from build123d import *

# Parameters (mm, degrees)
SKETCH3_W                = 100
SKETCH3_H                = 100
SKETCH3_W_2              = 80
SKETCH3_H_2              = 80
BOSS_EXTRUDE1_DEPTH      = 120
CUT_EXTRUDE6_DEPTH       = 186.47236991
CIRPATTERN1_COUNT        = 2
CIRPATTERN1_ANGLE        = 90
SKETCH19_R               = 13.375
SKETCH19_R_2             = 8.4375
BOSS_EXTRUDE3_DEPTH      = 10
BOSS_EXTRUDE4_START      = -110
SKETCH19_2_R             = 13.375
SKETCH19_2_R_2           = 8.4375
BOSS_EXTRUDE4_DEPTH      = 10
CUT_EXTRUDE4_DEPTH       = 186.47236991
CUT_EXTRUDE4_DEPTH_BACK  = 186.47236991
SKETCH8_R                = 8.4375
CUT_EXTRUDE11_START      = 120
SKETCH21_R               = 1.5
CUT_EXTRUDE11_DEPTH      = 10
CUT_EXTRUDE12_START      = 10
SKETCH21_2_R             = 1.5
CUT_EXTRUDE12_DEPTH      = 10
SKETCH9_W                = 10
SKETCH9_H                = 80
ELECTRONICSPLATE_DEPTH   = 120
CUT_EXTRUDE10_REACH      = 187.472
SKETCH18_W               = 80
SKETCH18_H               = 100
BEAGLEBONEHOLES_START    = 40
SKETCH12_R               = 1.7
BEAGLEBONEHOLES_DEPTH    = 10
RFDHOLES_START           = 40
SKETCH13_R               = 1.7
RFDHOLES_DEPTH           = 10
ANTENNACAVITY_START      = 30
SKETCH35_W               = 12
SKETCH35_H               = 43
ANTENNACAVITY_DEPTH      = 5
ZIPTIEHOLES_START        = 30
SKETCH36_W               = 3
SKETCH36_H               = 6.5
SKETCH36_W_2             = 6.5
SKETCH36_H_2             = 3
ZIPTIEHOLES_DEPTH        = 10
CUT_EXTRUDE16_START      = 30
SKETCH36_3_W             = 17
SKETCH36_3_H             = 6.5
SKETCH36_3_W_2           = 6.5
SKETCH36_3_H_2           = 15
CUT_EXTRUDE16_DEPTH      = 5
WIREHOLES_START          = 40
SKETCH37_W               = 10
SKETCH37_H               = 10
WIREHOLES_DEPTH          = 10
CUT_EXTRUDE17_DEPTH      = 186.47236991
CUT_EXTRUDE17_DEPTH_BACK = 186.47236991
SKETCH39_W               = 30
SKETCH39_H               = 100
SKETCH39_W_2             = 60
SKETCH39_W_3             = 10
SKETCH39_H_2             = 10


with BuildPart() as part:
    # Sketch3 → Boss-Extrude1 (new body)
    with BuildSketch(Plane(origin=(0, 0, 0), x_dir=(1, 0, 0), z_dir=(0, 1, 0))):
        with Locations((50, 50)):
            Rectangle(SKETCH3_W, SKETCH3_H)
        with Locations((50, 50)):
            Rectangle(SKETCH3_W_2, SKETCH3_H_2, mode=Mode.SUBTRACT)
    extrude(amount=BOSS_EXTRUDE1_DEPTH)

    # Sketch6 → Cut-Extrude6 (cut, symmetric)
    with BuildSketch(Plane.XY):
        Polygon((14.84187473, 110), (50, 67.810249676), (85.15812527, 110), align=None)
        Polygon((56.508541397, 60), (90, 100.189750324), (90, 19.810249676), align=None)
        Polygon((14.84187473, 10), (50, 52.189750324), (85.15812527, 10), align=None)
        Polygon((10, 19.810249676), (43.491458603, 60), (10, 100.189750324), align=None)
    cut_extrude6 = extrude(amount=CUT_EXTRUDE6_DEPTH, both=True, mode=Mode.SUBTRACT)

    # CirPattern1: Cut-Extrude6 ×2 about axis
    cirpattern1_axis = Axis((50, 0, -50), (0, 1, 0))
    for i in range(1, CIRPATTERN1_COUNT):
        add(cut_extrude6.rotate(cirpattern1_axis, i * CIRPATTERN1_ANGLE / (CIRPATTERN1_COUNT - 1)), mode=Mode.SUBTRACT)

    # Sketch19 → Boss-Extrude3 (add)
    # profile 1 of 4: a face of its own
    with BuildSketch(Plane(origin=(0, 120, 0), x_dir=(1, 0, 0), z_dir=(0, 1, 0))):
        with Locations((13.375, 86.625)):
            Circle(SKETCH19_R)
        with Locations((13.375, 86.625)):
            Circle(SKETCH19_R_2, mode=Mode.SUBTRACT)
    # profile 2 of 4: a face of its own
    with BuildSketch(Plane(origin=(0, 120, 0), x_dir=(1, 0, 0), z_dir=(0, 1, 0))):
        with Locations((86.625, 86.625)):
            Circle(SKETCH19_R)
        with Locations((86.625, 86.625)):
            Circle(SKETCH19_R_2, mode=Mode.SUBTRACT)
    # profile 3 of 4: a face of its own
    with BuildSketch(Plane(origin=(0, 120, 0), x_dir=(1, 0, 0), z_dir=(0, 1, 0))):
        with Locations((86.625, 13.375)):
            Circle(SKETCH19_R)
        with Locations((86.625, 13.375)):
            Circle(SKETCH19_R_2, mode=Mode.SUBTRACT)
    # profile 4 of 4: a face of its own
    with BuildSketch(Plane(origin=(0, 120, 0), x_dir=(1, 0, 0), z_dir=(0, 1, 0))):
        with Locations((13.375, 13.375)):
            Circle(SKETCH19_R)
        with Locations((13.375, 13.375)):
            Circle(SKETCH19_R_2, mode=Mode.SUBTRACT)
    extrude(amount=-BOSS_EXTRUDE3_DEPTH)

    # Sketch19<2> → Boss-Extrude4 (add)
    # profile 1 of 4: a face of its own
    with BuildSketch(Plane(origin=(0, 120, 0), x_dir=(1, 0, 0), z_dir=(0, 1, 0)).offset(BOSS_EXTRUDE4_START)):
        with Locations((13.375, 86.625)):
            Circle(SKETCH19_2_R)
    # profile 2 of 4: a face of its own
    with BuildSketch(Plane(origin=(0, 120, 0), x_dir=(1, 0, 0), z_dir=(0, 1, 0)).offset(BOSS_EXTRUDE4_START)):
        with Locations((86.625, 86.625)):
            Circle(SKETCH19_2_R)
        with Locations((86.625, 86.625)):
            Circle(SKETCH19_2_R_2, mode=Mode.SUBTRACT)
    # profile 3 of 4: a face of its own
    with BuildSketch(Plane(origin=(0, 120, 0), x_dir=(1, 0, 0), z_dir=(0, 1, 0)).offset(BOSS_EXTRUDE4_START)):
        with Locations((86.625, 13.375)):
            Circle(SKETCH19_2_R)
        with Locations((86.625, 13.375)):
            Circle(SKETCH19_2_R_2, mode=Mode.SUBTRACT)
    # profile 4 of 4: a face of its own
    with BuildSketch(Plane(origin=(0, 120, 0), x_dir=(1, 0, 0), z_dir=(0, 1, 0)).offset(BOSS_EXTRUDE4_START)):
        with Locations((13.375, 13.375)):
            Circle(SKETCH19_2_R)
        with Locations((13.375, 13.375)):
            Circle(SKETCH19_2_R_2, mode=Mode.SUBTRACT)
    extrude(amount=-BOSS_EXTRUDE4_DEPTH)

    # Sketch8 → Cut-Extrude4 (cut, two sides: drawn at the far end of the back side and taken through both)
    with BuildSketch(Plane(origin=(0, 0, 0), x_dir=(1, 0, 0), z_dir=(0, 1, 0)).offset(-CUT_EXTRUDE4_DEPTH_BACK)):
        with Locations(Location((13.375, 86.625, 0), (0, 0, 90))):
            Circle(SKETCH8_R)
        with Locations(Location((86.625, 86.625, 0), (0, 0, 90))):
            Circle(SKETCH8_R)
        with Locations(Location((13.375, 13.375, 0), (0, 0, 90))):
            Circle(SKETCH8_R)
        with Locations(Location((86.625, 13.375, 0), (0, 0, 90))):
            Circle(SKETCH8_R)
    extrude(amount=CUT_EXTRUDE4_DEPTH + CUT_EXTRUDE4_DEPTH_BACK, mode=Mode.SUBTRACT)

    # Sketch21 → Cut-Extrude11 (cut)
    with BuildSketch(Plane(origin=(0, 0, 0), x_dir=(1, 0, 0), z_dir=(0, 1, 0)).offset(CUT_EXTRUDE11_START)):
        with Locations(Location((5, 50, 0), (0, 0, 270))):
            Circle(SKETCH21_R)
        with Locations(Location((50, 95, 0), (0, 0, 270))):
            Circle(SKETCH21_R)
        with Locations(Location((95, 50, 0), (0, 0, 270))):
            Circle(SKETCH21_R)
        with Locations(Location((50, 5, 0), (0, 0, 270))):
            Circle(SKETCH21_R)
    extrude(amount=-CUT_EXTRUDE11_DEPTH, mode=Mode.SUBTRACT)

    # Sketch21<2> → Cut-Extrude12 (cut)
    with BuildSketch(Plane(origin=(0, 0, 0), x_dir=(1, 0, 0), z_dir=(0, 1, 0)).offset(CUT_EXTRUDE12_START)):
        with Locations(Location((5, 50, 0), (0, 0, 270))):
            Circle(SKETCH21_2_R)
        with Locations(Location((50, 95, 0), (0, 0, 270))):
            Circle(SKETCH21_2_R)
        with Locations(Location((95, 50, 0), (0, 0, 270))):
            Circle(SKETCH21_2_R)
        with Locations(Location((50, 5, 0), (0, 0, 270))):
            Circle(SKETCH21_2_R)
    extrude(amount=-CUT_EXTRUDE12_DEPTH, mode=Mode.SUBTRACT)

    # Sketch9 → ElectronicsPlate (add)
    with BuildSketch(Plane(origin=(0, 0, 0), x_dir=(1, 0, 0), z_dir=(0, 1, 0))):
        with Locations((35, 50)):
            Rectangle(SKETCH9_W, SKETCH9_H)
    extrude(amount=ELECTRONICSPLATE_DEPTH)

    # Sketch18 → Cut-Extrude10 (cut, up to next)
    with BuildSketch(Plane.ZY, mode=Mode.PRIVATE) as cut_extrude10_sk1:
        with Locations((-50, 60)):
            Rectangle(SKETCH18_W, SKETCH18_H)
    cut_extrude10_tool1 = extrude(cut_extrude10_sk1.sketch, amount=-CUT_EXTRUDE10_REACH, mode=Mode.PRIVATE) & part.part
    add(cut_extrude10_tool1.solids().sort_by_distance((0, 60, -50))[0], mode=Mode.SUBTRACT)

    # Sketch12 → BeagleboneHoles (cut)
    with BuildSketch(Plane(origin=(0, 0, 0), x_dir=(0, 0, -1), z_dir=(1, 0, 0)).offset(BEAGLEBONEHOLES_START)):
        with Locations((25.87, 41.96)):
            Circle(SKETCH12_R)
        with Locations((74.13, 41.96)):
            Circle(SKETCH12_R)
        with Locations((29.045, 108)):
            Circle(SKETCH12_R)
        with Locations((70.955, 108)):
            Circle(SKETCH12_R)
    extrude(amount=-BEAGLEBONEHOLES_DEPTH, mode=Mode.SUBTRACT)

    # Sketch13 → RFDHoles (cut)
    with BuildSketch(Plane(origin=(0, 0, 0), x_dir=(0, 0, -1), z_dir=(1, 0, 0)).offset(RFDHOLES_START)):
        with Locations((50, 30)):
            Circle(SKETCH13_R)
        with Locations((37.5, 67)):
            Circle(SKETCH13_R)
        with Locations((62.5, 67)):
            Circle(SKETCH13_R)
    extrude(amount=-RFDHOLES_DEPTH, mode=Mode.SUBTRACT)

    # Sketch35 → AntennaCavity (cut)
    with BuildSketch(Plane(origin=(0, 0, 0), x_dir=(0, 0, -1), z_dir=(1, 0, 0)).offset(ANTENNACAVITY_START)):
        with Locations((24, 68.5)):
            Rectangle(SKETCH35_W, SKETCH35_H)
        Polygon((18, 90), (30, 90), (50, 90), (50, 100), (18, 100), align=None)
        Polygon((50, 100), (50, 90), (70, 90), (82, 90), (82, 100), align=None)
        with Locations((76, 68.5)):
            Rectangle(SKETCH35_W, SKETCH35_H)
    extrude(amount=ANTENNACAVITY_DEPTH, mode=Mode.SUBTRACT)

    # Sketch36 → ZiptieHoles (cut)
    with BuildSketch(Plane(origin=(0, 0, 0), x_dir=(0, 0, -1), z_dir=(1, 0, 0)).offset(ZIPTIEHOLES_START)):
        with Locations((34, 53.701837694)):
            Rectangle(SKETCH36_W, SKETCH36_H)
        with Locations((14, 53.701837694)):
            Rectangle(SKETCH36_W, SKETCH36_H)
        with Locations((34, 76.513807116)):
            Rectangle(SKETCH36_W, SKETCH36_H)
        with Locations((14, 76.513807116)):
            Rectangle(SKETCH36_W, SKETCH36_H)
        with Locations((34.734232458, 86)):
            Rectangle(SKETCH36_W_2, SKETCH36_H_2)
        with Locations((34.734232458, 104)):
            Rectangle(SKETCH36_W_2, SKETCH36_H_2)
        with Locations((65.265767542, 104)):
            Rectangle(SKETCH36_W_2, SKETCH36_H_2)
        with Locations((65.265767542, 86)):
            Rectangle(SKETCH36_W_2, SKETCH36_H_2)
        with Locations((66, 76.513807116)):
            Rectangle(SKETCH36_W, SKETCH36_H)
        with Locations((86, 76.513807116)):
            Rectangle(SKETCH36_W, SKETCH36_H)
        with Locations((86, 53.701837694)):
            Rectangle(SKETCH36_W, SKETCH36_H)
        with Locations((66, 53.701837694)):
            Rectangle(SKETCH36_W, SKETCH36_H)
    extrude(amount=ZIPTIEHOLES_DEPTH, mode=Mode.SUBTRACT)

    # Sketch36<3> → Cut-Extrude16 (cut)
    with BuildSketch(Plane(origin=(0, 0, 0), x_dir=(0, 0, -1), z_dir=(1, 0, 0)).offset(CUT_EXTRUDE16_START)):
        with Locations((24, 76.513807116)):
            Rectangle(SKETCH36_3_W, SKETCH36_3_H)
        with Locations((34.734232458, 95)):
            Rectangle(SKETCH36_3_W_2, SKETCH36_3_H_2)
        with Locations((65.265767542, 95)):
            Rectangle(SKETCH36_3_W_2, SKETCH36_3_H_2)
        with Locations((76, 76.513807116)):
            Rectangle(SKETCH36_3_W, SKETCH36_3_H)
        with Locations((76, 53.701837694)):
            Rectangle(SKETCH36_3_W, SKETCH36_3_H)
        with Locations((24, 53.701837694)):
            Rectangle(SKETCH36_3_W, SKETCH36_3_H)
    extrude(amount=CUT_EXTRUDE16_DEPTH, mode=Mode.SUBTRACT)

    # Sketch37 → WireHoles (cut)
    with BuildSketch(Plane(origin=(0, 0, 0), x_dir=(0, 0, -1), z_dir=(1, 0, 0)).offset(WIREHOLES_START)):
        with Locations((45, 10)):
            Rectangle(SKETCH37_W, SKETCH37_H)
        with Locations((55, 10)):
            Rectangle(SKETCH37_W, SKETCH37_H)
        with Locations((55, 110)):
            Rectangle(SKETCH37_W, SKETCH37_H)
        with Locations((45, 110)):
            Rectangle(SKETCH37_W, SKETCH37_H)
    extrude(amount=-WIREHOLES_DEPTH, mode=Mode.SUBTRACT)

    # Sketch39 → Cut-Extrude17 (cut, two sides: drawn at the far end of the back side and taken through both)
    with BuildSketch(Plane(origin=(0, 0, 0), x_dir=(1, 0, 0), z_dir=(0, 1, 0)).offset(-CUT_EXTRUDE17_DEPTH_BACK)):
        with Locations((15, 50)):
            Rectangle(SKETCH39_W, SKETCH39_H)
        with Locations((70, 50)):
            Rectangle(SKETCH39_W_2, SKETCH39_H)
        with Locations((35, 95)):
            Rectangle(SKETCH39_W_3, SKETCH39_H_2)
        with Locations((35, 5)):
            Rectangle(SKETCH39_W_3, SKETCH39_H_2)
    extrude(amount=CUT_EXTRUDE17_DEPTH + CUT_EXTRUDE17_DEPTH_BACK, mode=Mode.SUBTRACT)


solid = part.part
Geometry check sheet. Reference: the model listing, model coordinates, mm. A direction names the side the tool comes from. Round coordinates to 2 decimals unless told otherwise and drop trailing zeros. Write each loop counter-clockwise with the first axis right and the second up, starting at its lowest first coordinate (ties: lowest second). Pieces come first, ordered by that corner, then holes. Notation, with made-up numbers: (43.25, 62) - (65.25, 62) arc R32 cw to (65.25, 95) - close; hole circle Ø11 at (-16.75, 74.5). An arc over 180 degrees is marked (long way). One line per item, written item: value.
1. Scan lines: L1, parallel to Z at x = 31.25, y = 88.5; L2, parallel to Z at x = 35.25, y = 67; L3, parallel to Y at x = 38, z = -57.5. Record each from-to range of solid material in increasing order.
The answers:
L1: z = -90 to -82, -70 to -68.52, -62.02 to -37.98, -31.48 to -30, -18 to -10
L2: z = -90 to -64.2, -60.8 to -39.2, -35.8 to -10
L3: y = 0 to 5, 15 to 105, 115 to 120
2. Set-up check for faces 1 (the face through (40, 59, -49)), 2 (the face through (37, 54, -32.5)), 3 (the face through (34, 56.952, -15)): record each of +Z, -Z, +X, -X, +Y, -Y from which the full face is reachable in a straight line by a thin tool's end or side.
The answers:
face 1: +Z, -Z, +X, +Y, -Y
face 2: +X, -X
face 3: -X
3. Mould release check, pull along Z, two halves, no side actions. Record for faces 4 (the face through (35, 59, -10)), 5 (the face through (35, 0, -51)), 6 (the face through (32, 49, -70)), 7 (the face through (34, 50.452, -67)): released by +Z, released by -Z, zero draft, split by the parting line, or undercut.
The answers:
face 4: released by +Z
face 5: zero draft
face 6: undercut
face 7: undercut
4. Cross-section at D-D on x = 31.75. Give the number of separate pieces and of enclosed holes in the cut face, and give its area (3 significant figures).
The answers:
separate pieces: 1
enclosed holes: 10
area: 7,040 mm^2
5. Cross-section at C-C on z = -50. Record the boundary of the cut face in (x, y), and give its area (3 significant figures).
The answers:
outline: (30, 0) - (40, 0) - (40, 5) - (30, 5) - close; (30, 15) - (40, 15) - (40, 28.3) - (30, 28.3) - close; (30, 31.7) - (40, 31.7) - (40, 105) - (30, 105) - (30, 100) - (35, 100) - (35, 90) - (30, 90) - close; (30, 115) - (40, 115) - (40, 120) - (30, 120) - close
area: 916 mm^2
6. Cross-section at A-A on y = 30. Record the boundary of the cut face in (x, z), and give its area (3 significant figures).
The answers:
outline: (30, -90) - (40, -90) - (40, -51.7) - (30, -51.7) - close; (30, -48.3) - (40, -48.3) - (40, -10) - (30, -10) - close
area: 766 mm^2
7. Cross-section at B-B on z = -25.87. Record the boundary of the cut face in (x, y).
The answers:
outline: (30, 0) - (40, 0) - (40, 40.26) - (30, 40.26) - close; (30, 43.66) - (40, 43.66) - (40, 120) - (30, 120) - (30, 100) - (35, 100) - (35, 47) - (30, 47) - close
